Part model, mm, in its own coordinate system. A direction names the side the tool comes from. Give positions to 0.01 mm unless a question says otherwise; leave off trailing zeros. Write each loop counter-clockwise with the first axis right and the second up, starting at its lowest first coordinate (ties: lowest second). Pieces come first, ordered by that corner, then holes. Notation, with made-up numbers: (-24.75, -32.5) - (10.25, -32.5) arc R28 cw to (10.25, -4.5) - close; hole circle Ø10 at (-33.75, -36.5). An arc over 180 degrees is marked (long way). Answer as a JSON object with one key per item and string values. Group by question number.
```python
from build123d import *

# Parameters (mm, degrees)
SKETCH1_W           = 93.99016
SKETCH1_H           = 50.8
BOSS_EXTRUDE1_DEPTH = 6.35
SKETCH2_W           = 6.35
SKETCH2_H           = 43.18
CUT_EXTRUDE1_DEPTH  = 6.35
SKETCH3_W           = 93.99016
SKETCH3_H           = 6.35
CUT_EXTRUDE2_DEPTH  = 2.54
SKETCH5_W           = 6.35
SKETCH5_H           = 6.35
CUT_EXTRUDE3_DEPTH  = 4.7625
SKETCH6_R           = 3.5
CUT_EXTRUDE4_DEPTH  = 6.35


with BuildPart() as part:
    # Sketch1 → Boss-Extrude1 (new body)
    with BuildSketch(Plane.XY):
        Rectangle(SKETCH1_W, SKETCH1_H)
    extrude(amount=BOSS_EXTRUDE1_DEPTH)

    # Sketch2 → Cut-Extrude1 (cut)
    with BuildSketch(Plane.XY.offset(6.35)):
        with Locations((-43.82008, -3.81)):
            Rectangle(SKETCH2_W, SKETCH2_H)
        with Locations((43.82008, -3.81)):
            Rectangle(SKETCH2_W, SKETCH2_H)
    extrude(amount=-CUT_EXTRUDE1_DEPTH, mode=Mode.SUBTRACT)

    # Sketch3 → Cut-Extrude2 (cut)
    with BuildSketch(Plane(origin=(0, 25.4, 0), x_dir=(1, 0, 0), z_dir=(0, 1, 0))):
        with Locations((0, -3.175)):
            Rectangle(SKETCH3_W, SKETCH3_H)
    extrude(amount=-CUT_EXTRUDE2_DEPTH, mode=Mode.SUBTRACT)

    # Sketch5 → Cut-Extrude3 (cut)
    with BuildSketch(Plane.ZY.offset(40.64508)):
        with Locations((3.175, 14.605)):
            Rectangle(SKETCH5_W, SKETCH5_H)
    cut_extrude3 = extrude(amount=-CUT_EXTRUDE3_DEPTH, mode=Mode.SUBTRACT)

    # Mirror1: Cut-Extrude3 across plane
    add(cut_extrude3.mirror(Plane(origin=(0, 0, 0), x_dir=(0, 0, 1), z_dir=(1, 0, 0))), mode=Mode.SUBTRACT)

    # Sketch6 → Cut-Extrude4 (cut)
    with BuildSketch(Plane.XY.offset(6.35)):
        with Locations((0.00592, -8.8499)):
            Circle(SKETCH6_R)
    extrude(amount=-CUT_EXTRUDE4_DEPTH, mode=Mode.SUBTRACT)


solid = part.part
```
1) Which spindle directions (+Z, -Z, +X, -X, +Y, -Y) get a long thin tool onto all of the face, cutting with end or side? Do faces 4 (the flat face through (40.645, -7, 3)), 5 (the flat face through (35.883, 15, 3)), 6 (the flat face through (-35.883, 15, 3)). Say none if no direction does.
2) Drop flat-ended pins along their axis: P1, Ø1.5, axis at y = -20.5, z = 1, coming from the -X side; P2, Ø5, axis at x = -20.5, y = -18.5, coming from the -Z side; P3, Ø3, axis at y = 13.5, z = 3, coming from the -X side; P4, Ø1.9, axis at y = 15.5, z = 4.5, coming from the +X side. Give the stop position or say it passes through.
3) Drill centre lines: line 1 along X through (y, z) = (16.5, 4.75); line 2 along X through (y, z) = (1, 0.5); line 3 along Y through (x, z) = (38.5, 2.25). Where is each one in solid material? Low to high. Write a range as from..to.
4) Saw through at A-A (y = -6.5). List the corners of the cut face in (x, z).
5) Two-plate mould, pull along Y, no slides. Class faces 1 (the flat face through (38, 11.43, 3)), 2 (the flat face through (-1, -25.4, 3)), 3 (the flat face through (46.995, 20, 3)): +Y half, -Y half, draft (parallel to the pull), parting line (faces both ways), or undercut.
6) Saw through at B-B (z = 4.5). List the corners of the cut face in (x, y).
7) Saw through at C-C (y = 7). List the corners of the cut face in (x, z), and give its area (3 significant figures).
Checks:
{
 "1": {"face 4": "+Z, -Z, +X, -Y", "face 5": "+Z, -Z, +X", "face 6": "+Z, -Z, -X"},
 "2": {"P1": "x = -40.65", "P2": "z = 0", "P3": "x = -35.88", "P4": "x = 35.88"},
 "3": {"line 1": "-35.88..35.88", "line 2": "-40.65..40.65", "line 3": "-25.4..11.43, 17.78..22.86"},
 "4": {"outline": "(-40.65, 0) - (-2.59, 0) - (-2.59, 6.35) - (-40.65, 6.35) - close; (2.6, 0) - (40.65, 0) - (40.65, 6.35) - (2.6, 6.35) - close"},
 "5": {"face 1": "undercut", "face 2": "-Y half", "face 3": "draft"},
 "6": {"outline": "(-47, 17.78) - (-35.88, 17.78) - (-35.88, 11.43) - (-40.65, 11.43) - (-40.65, -25.4) - (40.65, -25.4) - (40.65, 11.43) - (35.88, 11.43) - (35.88, 17.78) - (47, 17.78) - (47, 22.86) - (-47, 22.86) - close; hole circle Ø7 at (0.01, -8.85)"},
 "7": {"outline": "(-40.65, 0) - (40.65, 0) - (40.65, 6.35) - (-40.65, 6.35) - close", "area": "516 mm2"}
}
